Autodesk Inventor part; units mm, degrees
ref_plane "YZ Plane" through (0, 0, 0) normal (1, 0, 0) x (0, 1, 0)
ref_plane "XZ Plane" through (0, 0, 0) normal (0, 1, 0) x (-1, 0, 0)
ref_plane "XY Plane" through (0, 0, 0) normal (0, 0, 1) x (1, 0, 0)
sketch "Sketch1" plane through (0, 0, 0) normal (0, 0, 1) x (1, 0, 0)
  line L0 (0, 0) -> (181.174, 0)
  line L1 (181.174, 0) -> (181.174, 253.26)
  line L2 (181.174, 253.26) -> (0, 253.26)
  line L3 (0, 253.26) -> (0, 0)
  dimension "d0" = 181.174
  dimension "d1" = 253.26
extrude "Plate1" add sketch "Sketch1" along normal blind 0.5
sketch "Sketch2" plane through (181.174, 0, 0.5) normal (0, -1, 0) x (1, 0, 0)
  line L0 (-181.174, 0) -> (0, 0)
  line L1 (0, 0) -> (0, 10.195)
  line L2 (0, 10.195) -> (-181.174, 10.195)
  line L3 (-181.174, 10.195) -> (-181.174, 0)
edge flange "Flange1" height 10.695 angle 90 thickness 0.5 bend radius 0.5 thickness toward (0, -1, 0) relief tear relief width 0.5 relief depth 0.25 edges at (90.587, 0, 0.5) wall of the first edge with corners at (0, 0, 0.5) (181.174, 0, 0.5) (181.174, 0, 10.695) (0, 0, 10.695)
bend "Bend1"
corner "Corner1"
sketch "Sketch3" plane through (0, 0, 0.5) normal (0, 0, 1) x (1, 0, 0)
  line L0 (181.174, 253.26) -> (181.174, 0.5)
  line L1 (181.174, 253.26) -> (181.174, 168.36) construction
  line L2 (181.174, 168.36) -> (174.824, 168.36) construction
  line L3 (174.824, 168.36) -> (17.344, 168.36) construction
  line L4 (174.824, 168.36) -> (174.824, 13.48) construction
  circle A0 centre (174.824, 13.48) radius 1.5
  circle A1 centre (174.824, 168.36) radius 1.5
  circle A2 centre (17.344, 168.36) radius 1.5
  point P0 (0, 0)
  dimension "d13" = 84.9
  dimension "d14" = 6.35
  dimension "d15" = 157.48
  dimension "d16" = 154.88
  dimension "d17" = 3
  dimension "d18" = 3
  dimension "d19" = 3
extrude "Extrusion1" cut sketch "Sketch3" against normal blind 10
sketch "Sketch5" plane through (0, 0, 0.5) normal (0, 0, 1) x (1, 0, 0)
  circle A0 centre (17.344, 168.36) radius 1.5
  line L0 (17.344, 168.36) -> (17.344, 35.808) construction
  line L1 (17.344, 168.36) -> (149.896, 168.36) construction
  line L2 (17.344, 35.808) -> (17.344, 36.34) construction
  circle A1 centre (17.344, 36.34) radius 1.5
  point P0 (0, 0)
  dimension "d28" = 90
  dimension "d32" = 0.532
  dimension "d33" = 3
extrude "Extrusion4" cut sketch "Sketch5" against normal blind 10 contours A1
equation "\"d2\" = Thickness"
equation "\"d3\" = BendReliefWidth"
equation "\"d4\" = BendReliefDepth"
equation "\"d5\" = MinimumRemnant"
equation "\"d6\" = TransitionRadius"
equation "\"d9\" = BendRadius"
equation "\"d10\" = CornerReliefSize"
equation "\"d11\" = GapSize"
equation "\"d12\" = JacobiRadiusSize"
equation "\"BendRadius\" = Thickness"
equation "\"BendReliefWidth\" = Thickness"
equation "\"BendReliefDepth\" = 0.5 * Thickness"
equation "\"CornerReliefSize\" = 4 * Thickness"
equation "\"MinimumRemnant\" = 2 * Thickness"
equation "\"TransitionRadius\" = BendRadius"
equation "\"JacobiRadiusSize\" = BendRadius"
equation "\"GapSize\" = Thickness"
properties part number "dads trunk"
Design review of the part built by this model. Coordinates are the model's own, in mm. A direction names the side the tool comes from. Coordinates: 2 decimals unless noted, no trailing zeros. Write each loop counter-clockwise with the first axis right and the second up, starting at its lowest first coordinate (ties: lowest second). Pieces come first, ordered by that corner, then holes.
1) Add section C-C (y = 83). Write out the cut boundary in (x, z), plus the area to 3 significant figures.
2) Machinability: for faces 1 (the flat face through (89, 129, 0.5)), 2 (the flat face through (92, -0.5, 6)), which of the approach directions +Z, -Z, +X, -X, +Y, -Y give a long, thin tool a straight path to every point of the face, cutting with its end or side? Answer none if there is none.
3) To check wall thickness, follow L1, parallel to X at y = 168.36, z = 0.25; L2, parallel to Z at x = 32.5, y = 157; L3, parallel to Y at x = 107, z = 7. State the ranges of each line that lie inside material, in increasing order.
4) Add section B-B (z = 4). Write out the cut boundary in (x, y), plus the area to 3 significant figures.
5) Insertion check: pin 1 (1 mm diameter, centred on x = 83, z = 5.5, fed in from +Y); pin 2 (3.5 mm diameter, centred on x = 174.824, y = 13.48, fed in from +Z). Each pin has a flat end and moves straight along its axis. Give the tip position at first contact, or say it passes through.
6) Add section A-A (x = 50.5). Write out the cut boundary in (y, z) (3 decimals), plus the area to 3 significant figures.
Check result:
1. outline: (0, 0) - (181.17, 0) - (181.17, 0.5) - (0, 0.5) - close
1. area: 90.6 mm2
2. face 1: +Z, +X, -X, +Y
2. face 2: +Z, -Z, +X, -X, -Y
3. L1: x = 0 to 15.84, 18.84 to 173.32, 176.32 to 181.17
3. L2: z = 0 to 0.5
3. L3: y = -0.5 to 0
4. outline: (0, -0.5) - (181.17, -0.5) - (181.17, 0) - (0, 0) - close
4. area: 90.6 mm2
5. pin 1: stops at y = 0
5. pin 2: stops at z = 0.5
6. outline: (-0.5, 1) arc R1 ccw to (0.5, 0) - (253.26, 0) - (253.26, 0.5) - (0.5, 0.5) arc R0.5 cw to (0, 1) - (0, 10.695) - (-0.5, 10.695) - close
6. area: 132 mm2
